```python
from build123d import *

# Parameters (mm, degrees)
SKETCH_1_R      = 1.6
EXTRUDE_1_DEPTH = 1.6
FILLET_1_R      = 2


with BuildPart() as part:
    # 草图1 → 凸台-拉伸1 (new body)
    with BuildSketch(Plane.XY):
        Polygon((8.5, 2.2), (8.5, -16.15), (-21.5, -16.15), (-21.5, -36.15), (8.5, -36.15), (8.5, -50), (-50, -50), (-50, -2.2), (-8.5, -2.2), (-8.5, 16.15), (21.5, 16.15), (21.5, 36.15), (-8.5, 36.15), (-8.5, 50), (50, 50), (50, 2.2), align=None)
        with Locations((-45, -36.25)):
            Circle(SKETCH_1_R, mode=Mode.SUBTRACT)
        with Locations((-45, -16.25)):
            Circle(SKETCH_1_R, mode=Mode.SUBTRACT)
        with Locations((45, 16.25)):
            Circle(SKETCH_1_R, mode=Mode.SUBTRACT)
        with Locations((45, 36.25)):
            Circle(SKETCH_1_R, mode=Mode.SUBTRACT)
    extrude(amount=EXTRUDE_1_DEPTH)

    # 圆角1
    fillet_1_edges = [part.edges().sort_by_distance(p)[0] for p in [
        (8.5, 2.2, 0.8),
        (8.5, -16.15, 0.8),
        (-21.5, -16.15, 0.8),
        (-21.5, -36.15, 0.8),
        (8.5, -36.15, 0.8),
        (8.5, -50, 0.8),
        (-50, -50, 0.8),
        (-50, -2.2, 0.8),
        (-8.5, -2.2, 0.8),
        (-8.5, 16.15, 0.8),
        (21.5, 16.15, 0.8),
        (21.5, 36.15, 0.8),
        (-8.5, 36.15, 0.8),
        (-8.5, 50, 0.8),
        (50, 50, 0.8),
        (50, 2.2, 0.8),
    ]]
    fillet(fillet_1_edges, radius=FILLET_1_R)


solid = part.part
```
Could you check a few things on this model? Use its own coordinates, in mm. Give positions to 0.01 mm unless a question says otherwise; leave off trailing zeros. Write each loop counter-clockwise with the first axis right and the second up, starting at its lowest first coordinate (ties: lowest second). Pieces come first, ordered by that corner, then holes. Notation, with made-up numbers: (-12, 1) -> (41, 1) arc R19 ccw to (41, 10) -> close; hole circle Ø7 at (57, 48.5). An arc over 180 degrees is marked (long way). Write each question's results on one line, items separated by ' | '.
1. Will these pins go through, and if not, where does the flat tip stop? pin 1 Ø0.8 at (y, z) = (8.5, 1) entering from -X; pin 2 Ø0.8 at (y, z) = (-8, 1) entering from +X; pin 3 Ø0.5 at (y, z) = (-29, 0.5) entering from +X; pin 4 Ø3 at (x, y) = (45, 36.25) entering from -Z.
Check sheet entries:
pin 1: stops at x = -8.5 | pin 2: stops at x = 8.5 | pin 3: stops at x = -21.5 | pin 4: passes through
2. I want a section at B-B, the plane x = 13. Write out the boundary of the cut face in (y, z), then the cut area to 3 significant figures.
Check sheet entries:
outline: (2.2, 0) -> (16.15, 0) -> (16.15, 1.6) -> (2.2, 1.6) -> close; (36.15, 0) -> (50, 0) -> (50, 1.6) -> (36.15, 1.6) -> close | area: 44.5 mm²
3. I need wall thicknesses on L1, parallel to Y at x = -45, z = 1.3; L2, parallel to Y at x = 1.5, z = 0.7; L3, parallel to Y at x = -12, z = 0.7. Which ranges of each line are inside material? Lowest first, please.
Check sheet entries:
L1: y = -50 to -37.85, -34.65 to -17.85, -14.65 to -2.2 | L2: y = -50 to -36.15, -16.15 to 16.15, 36.15 to 50 | L3: y = -50 to -36.15, -16.15 to -2.2
4. If we mould it in two halves opening along X, with no side actions, what happens to faces 1 (the cylindrical face through (44.792, 17.836, 0.789)), 2 (the flat face through (1, 1, 0))? For each: released by +X, released by -X, zero draft, split by the parting line, or undercut.
Check sheet entries:
face 1: undercut | face 2: zero draft
5. I want a section at C-C, the plane z = 1.25. Count the separate pieces of the cut face and the enclosed holes in it, then the cut area to 3 significant figures.
Check sheet entries:
separate pieces: 1 | enclosed holes: 4 | area: 4,430 mm²
6. I want a section at A-A, the plane x = -45. Write out the boundary of the cut face in (y, z), then the cut area to 3 significant figures.
Check sheet entries:
outline: (-50, 0) -> (-37.85, 0) -> (-37.85, 1.6) -> (-50, 1.6) -> close; (-34.65, 0) -> (-17.85, 0) -> (-17.85, 1.6) -> (-34.65, 1.6) -> close; (-14.65, 0) -> (-2.2, 0) -> (-2.2, 1.6) -> (-14.65, 1.6) -> close | area: 66.2 mm²
7. I want a section at D-D, the plane y = 31.5. Write out the boundary of the cut face in (x, z).
Check sheet entries:
outline: (21.5, 0) -> (50, 0) -> (50, 1.6) -> (21.5, 1.6) -> close
